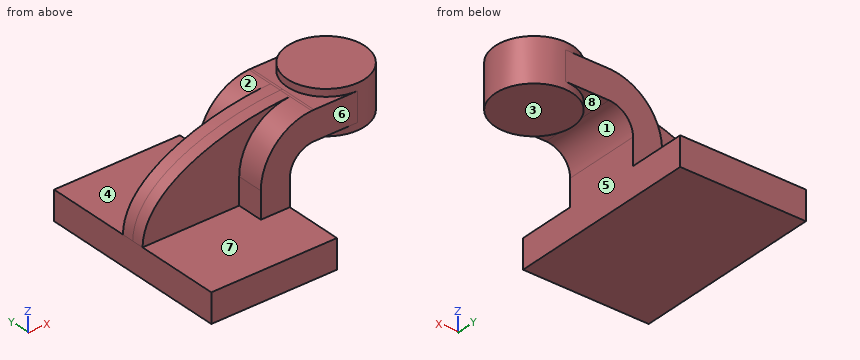
from build123d import *

# Parameters (mm, degrees)
F1_DEPTH = 63.5
F2_DEPTH = 25.4
F0_W     = 25.4
F0_H     = 19.05
F3_DEPTH = 25.4
F4_DEPTH = 7.9375


with BuildPart() as f1:
    # F0 (on Front) → F1 (new body, symmetric)
    with BuildSketch(Plane.XZ):
        Polygon((-41.275, 9.525), (-41.275, -9.525), (41.275, -9.525), (41.275, 9.525), (22.225, 9.525), align=None)
    extrude(amount=F1_DEPTH, both=True)

    # F0 (on Front) → F2 (join, symmetric)
    with BuildSketch(Plane.XZ):
        with BuildLine():
            Line((22.225, 9.525), (41.275, 9.525))
            Line((41.275, 9.525), (41.275, 27.0002))
            ThreePointArc((41.275, 27.0002), (45.9246798487, 38.2255201513), (57.15, 42.8752))
            Line((57.15, 42.8752), (60.325, 42.8752))
            Line((60.325, 42.8752), (60.325, 61.9252))
            Line((60.325, 61.9252), (57.15, 61.9252))
            add(Edge.make_bspline(
                [(55.6487642721, 61.8929201045), (56.1526188138, 61.9062395272), (56.6530888928, 61.9169959284), (57.15, 61.9252)],
                knots=[110.0594590217, 110.0594590217, 110.0594590217, 110.0594590217, 111.5045361635, 111.5045361635, 111.5045361635, 111.5045361635], degree=3))
            ThreePointArc((55.6487642721, 61.8929201045), (31.9291129934, 51.1593076739), (22.225, 27.0002))
            Line((22.225, 27.0002), (22.225, 9.525))
        make_face()
    extrude(amount=F2_DEPTH, both=True)

    # F0 (on Front) → F3 (join, symmetric)
    with BuildSketch(Plane.XZ):
        with Locations((73.025, 52.4002)):
            Rectangle(F0_W, F0_H)
    extrude(amount=F3_DEPTH, both=True)

    # F0 (on Front) → F4 (join, symmetric)
    with BuildSketch(Plane.XZ):
        with BuildLine():
            add(Edge.make_bspline(
                [(-41.275, 9.525), (-40.7319258576, 44.9970073135), (17.2743711817, 60.8784908984), (55.6487642721, 61.8929201045)],
                knots=[0, 0, 0, 0, 110.0594590217, 110.0594590217, 110.0594590217, 110.0594590217], degree=3))
            Line((-41.275, 9.525), (22.225, 9.525))
            Line((22.225, 9.525), (22.225, 27.0002))
            ThreePointArc((22.225, 27.0002), (31.9291129934, 51.1593076739), (55.6487642721, 61.8929201045))
        make_face()
    extrude(amount=F4_DEPTH, both=True)

    # F0 (on Front) → F5 (revolve)
    with BuildSketch(Plane.XZ):
        Polygon((85.725, 66.675), (85.725, 61.9252), (85.725, 42.8752), (85.725, 38.1), (111.125, 38.1), (111.125, 66.675), align=None)
    revolve(axis=Axis((85.725, 0, 52.3875), (0, 0, 1)))


solid = f1.part
Work out the finished part from the listing and answer in its coordinate system (mm). Face numbers are marked on the shaded views. A direction names the side the tool comes from. Coordinates: 2 decimals unless noted, no trailing zeros. Loops run counter-clockwise (first coordinate to the right, second up) from the corner with the lowest first, then second, coordinate; pieces in that order, holes last. Notation, with made-up numbers: M 55,71 L 71,71 A13 ccw 71,95 Z; hole C 22,-26.75 d4. An arc over 180 degrees is marked long. Answer in a Markdown table with one row per item. Add a question column.
1. A tool of negligible diameter and unlimited length cuts with its end or side. For the marked faces 4, 5, 6, 7 and 8, from which of +Z, -Z, +X, -X, +Y, -Y can it reach the whole face along a straight path? Write none if from no direction.
2. Flat-ended cylindrical pins translate along their axes: P1, Ø14, axis at y = -20.5, z = 20.5, coming from the -X side (3 decimals); P2, Ø15.5, axis at x = 1.5, z = 40.5, coming from the -Y side; P3, Ø2, axis at y = -9.5, z = 42.5, coming from the -X side. Find the tip coordinate at first contact, or state that the pin passes through.
3. Find section B-B, the plane y = 29. Write down the section's boundary in (x, z) (3 decimals), then the cut area to 3 significant figures.
4. Consider L1, parallel to Y at x = -15.5, z = 39; L2, parallel to X at y = -6.5, z = 9.5 (3 decimals); L3, parallel to Y at x = 63.5, z = 56. Determine where each line is inside the solid, lowest interval first.
5. Find section C-C, the plane x = 91. Write down the section's boundary in (y, z) (3 decimals), then the cut area to 3 significant figures.
6. The mould has two halves that part along X. Classify the marked faces 1, 2 and 3: pulls with the +X half, pulls with the -X half, needs draft (parallel to the pull), parting line crosses it, or undercut.
7. Find section A-A, the plane x = 62.5. Write down the section's boundary in (y, z) (3 decimals), then the cut area to 3 significant figures.
Reported:
| question | item | result |
|---|---|---|
| 1 | face 4 | +Z, -X, +Y |
| 1 | face 5 | -Z, +X, +Y, -Y |
| 1 | face 6 | +Z, +X, -X, -Y |
| 1 | face 7 | +Z, -X, -Y |
| 1 | face 8 | -Z |
| 2 | P1 | stops at x = 22.225 |
| 2 | P2 | stops at y = -7.94 |
| 2 | P3 | stops at x = 25.38 |
| 3 | outline | M -41.275,-9.525 L 41.275,-9.525 L 41.275,9.525 L -41.275,9.525 Z |
| 3 | area | 1,570 mm^2 |
| 4 | L1 | y = -7.94 to 7.94 |
| 4 | L2 | x = -41.275 to 41.275 |
| 4 | L3 | y = -25.4 to 25.4 |
| 5 | outline | M -24.846,38.1 L 24.846,38.1 L 24.846,66.675 L -24.846,66.675 Z |
| 5 | area | 1,420 mm^2 |
| 6 | face 1 | undercut |
| 6 | face 2 | pulls with the -X half |
| 6 | face 3 | needs draft |
| 7 | outline | M -25.4,42.875 L -10.284,42.875 L -10.284,38.1 L 10.284,38.1 L 10.284,42.875 L 25.4,42.875 L 25.4,61.925 L 10.284,61.925 L 10.284,66.675 L -10.284,66.675 L -10.284,61.925 L -25.4,61.925 Z |
| 7 | area | 1,160 mm^2 |
